from build123d import *

# Parameters (mm, degrees)
SKETCH1_W                = 100
SKETCH1_H                = 100
BOSS_EXTRUDE1_DEPTH      = 327.8
SKETCH2_W                = 8.5
SKETCH2_H                = 8.5
BOSS_EXTRUDE2_DEPTH      = 6.5
CHAMFER1_SIZE            = 1
SKETCH3_R                = 32
BOSS_EXTRUDE3_DEPTH      = 36
CHAMFER1_OF_MIRROR1_SIZE = 1
FILLET1_R                = 1
SKETCH6_W                = 83
SKETCH6_H                = 327.8
CUT_EXTRUDE1_DEPTH       = 2
CIRPATTERN1_COUNT        = 4
FILLET2_R                = 1
FILLET3_R                = 1
CHAMFER2_SIZE            = 1


with BuildPart() as part:
    # Sketch1 → Boss-Extrude1 (new body)
    with BuildSketch(Plane(origin=(0, 0, 0), x_dir=(1, 0, 0), z_dir=(0, 1, 0))):
        Rectangle(SKETCH1_W, SKETCH1_H)
    extrude(amount=BOSS_EXTRUDE1_DEPTH)

    # Sketch2 → Boss-Extrude2 (add)
    with BuildSketch(Plane(origin=(0, 327.8, 0), x_dir=(1, 0, 0), z_dir=(0, 1, 0))):
        with Locations((45.75, 45.75)):
            Rectangle(SKETCH2_W, SKETCH2_H)
        with Locations((-45.75, 45.75)):
            Rectangle(SKETCH2_W, SKETCH2_H)
        with Locations((45.75, -45.75)):
            Rectangle(SKETCH2_W, SKETCH2_H)
        with Locations((-45.75, -45.75)):
            Rectangle(SKETCH2_W, SKETCH2_H)
    boss_extrude2 = extrude(amount=BOSS_EXTRUDE2_DEPTH)

    # Chamfer1
    chamfer1_edges = [part.edges().sort_by_distance(p)[0] for p in [
        (45.75, 334.3, -41.5),
        (41.5, 334.3, -45.75),
        (45.75, 334.3, -50),
        (50, 334.3, -45.75),
        (41.5, 334.3, 45.75),
        (45.75, 334.3, 41.5),
        (50, 334.3, 45.75),
        (45.75, 334.3, 50),
        (-50, 334.3, 45.75),
        (-45.75, 334.3, 41.5),
        (-41.5, 334.3, 45.75),
        (-45.75, 334.3, 50),
        (-45.75, 334.3, -50),
        (-41.5, 334.3, -45.75),
        (-45.75, 334.3, -41.5),
        (-50, 334.3, -45.75),
    ]]
    chamfer(chamfer1_edges, length=CHAMFER1_SIZE)

    # Sketch3 → Boss-Extrude3 (add)
    with BuildSketch(Plane(origin=(0, 327.8, 0), x_dir=(1, 0, 0), z_dir=(0, 1, 0))):
        with Locations(Location((0, 0, 0), (0, 0, 90))):
            Circle(SKETCH3_R)
    extrude(amount=BOSS_EXTRUDE3_DEPTH)

    # Mirror1: Boss-Extrude2 across plane
    add(boss_extrude2.mirror(Plane.ZX.offset(163.9)))

    # Chamfer1 of Mirror1
    chamfer1_of_mirror1_edges = [part.edges().sort_by_distance(p)[0] for p in [
        (45.75, -6.5, -41.5),
        (41.5, -6.5, -45.75),
        (45.75, -6.5, -50),
        (50, -6.5, -45.75),
        (41.5, -6.5, 45.75),
        (45.75, -6.5, 41.5),
        (50, -6.5, 45.75),
        (45.75, -6.5, 50),
        (-50, -6.5, 45.75),
        (-45.75, -6.5, 41.5),
        (-41.5, -6.5, 45.75),
        (-45.75, -6.5, 50),
        (-45.75, -6.5, -50),
        (-41.5, -6.5, -45.75),
        (-45.75, -6.5, -41.5),
        (-50, -6.5, -45.75),
    ]]
    chamfer(chamfer1_of_mirror1_edges, length=CHAMFER1_OF_MIRROR1_SIZE)

    # Fillet1
    fillet1_edges = [part.edges().sort_by_distance(p)[0] for p in [
        (-50, 163.9, -50),
        (50, 163.9, -50),
        (50, 163.9, 50),
        (-50, 163.9, 50),
    ]]
    fillet(fillet1_edges, radius=FILLET1_R)

    # Sketch6 → Cut-Extrude1 (cut)
    with BuildSketch(Plane(origin=(0, 0, -50), x_dir=(-1, 0, 0), z_dir=(0, 0, -1))):
        with Locations((0, 163.9)):
            Rectangle(SKETCH6_W, SKETCH6_H)
    cut_extrude1 = extrude(amount=-CUT_EXTRUDE1_DEPTH, mode=Mode.SUBTRACT)

    # CirPattern1: Cut-Extrude1 ×4 about axis
    cirpattern1_axis = Axis((0, 0, 0), (0, 1, 0))
    for i in range(1, CIRPATTERN1_COUNT):
        add(cut_extrude1.rotate(cirpattern1_axis, i * 360 / CIRPATTERN1_COUNT), mode=Mode.SUBTRACT)

    # Fillet2
    fillet2_edges = [part.edges().sort_by_distance(p)[0] for p in [
        (0, 363.8, 32),
    ]]
    fillet(fillet2_edges, radius=FILLET2_R)

    # Fillet3
    fillet3_edges = [part.edges().sort_by_distance(p)[0] for p in [
        (41.5, -2.75, -41.5),
        (41.5, -2.75, 41.5),
        (-41.5, -2.75, 41.5),
        (-41.5, -2.75, -41.5),
        (50, 163.9, -41.5),
        (41.5, 330.55, -41.5),
        (41.5, 163.9, -50),
        (-41.5, 163.9, -50),
        (50, 163.9, 41.5),
        (41.5, 163.9, 50),
        (41.5, 330.55, 41.5),
        (-41.5, 163.9, 50),
        (-50, 163.9, 41.5),
        (-50, 163.9, -41.5),
        (-41.5, 330.55, 41.5),
        (-41.5, 330.55, -41.5),
    ]]
    fillet(fillet3_edges, radius=FILLET3_R)

    # Chamfer2
    chamfer2_edges = [part.edges().sort_by_distance(p)[0] for p in [
        (48, 0, 0),
        (0, 0, 48),
        (0, 0, -48),
        (-48, 0, 0),
        (48, 327.8, 0),
        (0, 327.8, -48),
        (0, 327.8, 48),
        (-48, 327.8, 0),
    ]]
    chamfer(chamfer2_edges, length=CHAMFER2_SIZE)


solid = part.part
Work out the finished part from the listing and answer in its coordinate system (mm). A direction names the side the tool comes from. Round coordinates to 2 decimals unless told otherwise and drop trailing zeros. Write each loop counter-clockwise with the first axis right and the second up, starting at its lowest first coordinate (ties: lowest second). Pieces come first, ordered by that corner, then holes. Notation, with made-up numbers: (5, 17.5) -> (47, 17.5) arc R30 ccw to (47, 53.5) -> close; hole circle Ø1 at (-26.5, -11). An arc over 180 degrees is marked (long way). Answer as CSV lines item,"result". Start each with the question number.
(1) A tool of negligible diameter and unlimited length cuts with its end or side. For faces 1 (the flat face through (-46, 334.3, 46)), 2 (the flat face through (48, 166, 1)), from which of +Z, -Z, +X, -X, +Y, -Y can it reach the whole face along a straight path? Write none if from no direction.
(2) Each of these flat-tipped pins is pushed along its axis until it touches: pin 1 (1 mm diameter, centred on y = 139.5, z = 36, fed in from -X); pin 2 (5 mm diameter, centred on x = -12, z = 24, fed in from -Y); pin 3 (1 mm diameter, centred on y = 234.5, z = 14, fed in from +X). Where does it stop, or does it pass through?
(3) The mould has two halves that part along X. Classify faces 3 (the flat face through (50, 166, -46)), 4 (the flat face through (48.4, 189.8, -41.5)), 5 (the flat face through (-1, 166, 48)), 6 (the flat face through (-48, 166, -1)): +X half, -X half, draft (parallel to the pull), parting line (faces both ways), or undercut.
(4) Find the intervals of material crossed by probe 1 along X at (y, z) = (119, -31); probe 2 along Y at (x, z) = (-24.5, -33.5), in increasing order.
(5) The part is cut by section B-B, the plane z = 0. Give the vertices of the cut face in (x, y), then the cut area to 3 significant figures.
(6) The part is cut by section C-C, the plane x = 0. Give the vertices of the cut face in (y, z), then the cut area to 3 significant figures.
(7) The part is cut by section D-D, the plane z = 37.5. Give the vertices of the cut face in (x, y), then the cut area to 3 significant figures.
Output values:
1,face 1,"+Z, -Z, +X, -X, +Y"
1,face 2,"+X, +Y, -Y"
2,pin 1,"stops at x = -48"
2,pin 2,"stops at y = 0"
2,pin 3,"stops at x = 48"
3,face 3,"+X half"
3,face 4,"draft"
3,face 5,"undercut"
3,face 6,"-X half"
4,probe 1,"x = -48 to 48"
4,probe 2,"y = 0 to 327.8"
5,outline,"(-48, 1) -> (-47, 0) -> (47, 0) -> (48, 1) -> (48, 326.8) -> (47, 327.8) -> (32, 327.8) -> (32, 362.8) arc R1 ccw to (31, 363.8) -> (-31, 363.8) arc R1 ccw to (-32, 362.8) -> (-32, 327.8) -> (-47, 327.8) -> (-48, 326.8) -> close"
5,area,"33,800 mm²"
6,outline,"(0, -47) -> (1, -48) -> (326.8, -48) -> (327.8, -47) -> (327.8, -32) -> (362.8, -32) arc R1 ccw to (363.8, -31) -> (363.8, 31) arc R1 ccw to (362.8, 32) -> (327.8, 32) -> (327.8, 47) -> (326.8, 48) -> (1, 48) -> (0, 47) -> close"
6,area,"33,800 mm²"
7,outline,"(-48, 1) -> (-47, 0) -> (47, 0) -> (48, 1) -> (48, 326.8) -> (47, 327.8) -> (-47, 327.8) -> (-48, 326.8) -> close"
7,area,"31,500 mm²"
